from build123d import *

# Parameters (mm, degrees)
CYLINDER116_R     = 1.2
CYLINDER116_DEPTH = 100
FILLET007_R       = 1
FILLET008_R       = 1


with BuildPart() as obj1:
    # Cylinder116 → Cylinder116 (new body)
    with BuildSketch(Plane.XY.offset(-50)):
        Circle(CYLINDER116_R)
    extrude(amount=CYLINDER116_DEPTH)


with BuildPart() as obj2:
    # Cone004 → Cone004 (revolve)
    with BuildSketch(Plane(origin=(0, 0, -3), x_dir=(1, 0, 0), z_dir=(0, -1, 0))):
        Polygon((0, 0), (1.2, 0), (2, 3), (0, 3), align=None)
    revolve(axis=Axis((0, 0, -3), (0, 0, 1)))


with BuildPart() as syringe_tip_hole_fusion:
    # Cone → Cone (revolve)
    with BuildSketch(Plane.XZ):
        Polygon((0, 0), (2, 0), (2.2, 6.6), (0, 6.6), align=None)
    revolve(axis=Axis((0, 0, 0), (0, 0, 1)))

    # Fusion017: union obj1, obj2
    add(obj1.part)
    add(obj2.part)


with BuildPart() as obj3:
    # Cone003 → Cone003 (revolve)
    with BuildSketch(Plane(origin=(0, 0, -3), x_dir=(1, 0, 0), z_dir=(0, -1, 0))):
        Polygon((0, 0), (2.1, 0), (4, 3), (0, 3), align=None)
    revolve(axis=Axis((0, 0, -3), (0, 0, 1)))


with BuildPart() as obj4:
    # Cone002 → Cone002 (revolve)
    with BuildSketch(Plane(origin=(0, 0, -13), x_dir=(1, 0, 0), z_dir=(0, -1, 0))):
        Polygon((0, 0), (1.6, 0), (2.1, 10), (0, 10), align=None)
    revolve(axis=Axis((0, 0, -13), (0, 0, 1)))

    # Fillet007
    fillet007_edges = [obj4.edges().sort_by_distance(p)[0] for p in [
        (-1.6, 0, -13),
    ]]
    fillet(fillet007_edges, radius=FILLET007_R)


with BuildPart() as syringe_tip_cut_fillet:
    # Cone001 → Cone001 (revolve)
    with BuildSketch(Plane.XZ):
        Polygon((0, 0), (4, 0), (4.2, 6.6), (0, 6.6), align=None)
    revolve(axis=Axis((0, 0, 0), (0, 0, 1)))

    # Fusion016: union obj3, obj4
    add(obj3.part)
    add(obj4.part)

    # Cut012: cut syringe tip hole fusion
    add(syringe_tip_hole_fusion.part, mode=Mode.SUBTRACT)

    # Fillet008
    fillet008_edges = [syringe_tip_cut_fillet.edges().sort_by_distance(p)[0] for p in [
        (-2.2, 0, 6.6),
    ]]
    fillet(fillet008_edges, radius=FILLET008_R)


solid = syringe_tip_cut_fillet.part
Work out the finished part from the listing and answer in its coordinate system (mm). Give positions to 0.01 mm unless a question says otherwise; leave off trailing zeros. Write each loop counter-clockwise with the first axis right and the second up, starting at its lowest first coordinate (ties: lowest second). Pieces come first, ordered by that corner, then holes.
Q1. Straight lines are drawn through the part: L1, parallel to X at y = 0, z = -5; L2, parallel to Y at x = 0, z = -6.25; L3, parallel to X at y = 0, z = -6.5 (3 decimals). For each, find the intervals that lie inside material, in ascending order.
Answer:
L1: x = -2 to -1.2, 1.2 to 2
L2: y = -1.94 to -1.2, 1.2 to 1.94
L3: x = -1.925 to -1.2, 1.2 to 1.925
Q2. The part is cut by section B-B on z = -7. Give the vertices of the cut face in (x, y).
Answer:
outline: circle Ø3.8 at (0, 0); hole circle Ø2.4 at (0, 0)
Q3. The part is cut by section A-A on z = -5. Give the vertices of the cut face in (x, y).
Answer:
outline: circle Ø4 at (0, 0); hole circle Ø2.4 at (0, 0)
Q4. Given pin 1 (2 mm diameter, centred on y = -2, z = 0.5, fed in from +X); pin 2 (5 mm diameter, centred on x = -0.5, z = -7.5, fed in from -Y); pin 3 (4 mm diameter, centred on y = 2, z = -0.5, fed in from -X), each flat-ended and moving along its own axis, determine where each tip first touches the part or whether it passes through.
Answer:
pin 1: stops at x = 3.89
pin 2: stops at y = -2
pin 3: stops at x = -4.01
Q5. For a pull along Y with two mould halves and no side action, classify faces 1 (the face through (0.65, 1.01, -7.99)), 2 (the face through (-0.9, -4, 3.3)), 3 (the face through (-1.656, -1.27, 2.855)), 4 (the face through (-2, 3, 6.6)) as released by +Y, released by -Y, zero draft, split by the parting line, or undercut.
Answer:
face 1: undercut
face 2: split by the parting line
face 3: undercut
face 4: zero draft
